Verification items for the finished model (mm, model axes). Round coordinates to 2 decimals unless told otherwise and drop trailing zeros. Order: outer loops, then holes, each group sorted by start corner. A loop starts at its lowest first (then second) coordinate and runs counter-clockwise, first axis right, second up. Notation, with made-up numbers: (36, -18) -> (78, -18) arc R22 cw to (78, 20) -> close; hole circle Ø10 at (88.25, -34). An arc over 180 degrees is marked (long way). Return JSON: item names as keys, results as strings. Group by question number.
Item 1: Draft check along Y on faces 1 (the flat face through (9, 0, 9)), 2 (the cylindrical face through (8.628, 7.255, 8.124)), 3 (the flat face through (0, 11, 9)). Enter one of: pulls with the +Y half, pulls with the -Y half, needs draft (parallel to the pull), parting line crosses it, or undercut.
Item 2: Sectioned sample at C-C on y = 6. Record the cut outline in (x, z).
Item 3: Depth check by flat-ended pin: pin 1 Ø8 at (x, y) = (8, 5) entering from -Z; pin 2 Ø3 at (y, z) = (8.78, 8.76) entering from -X. Enter the tip coordinate at first touch or a pass-through.
Item 4: Sectioned sample at B-B on x = 7.25. Record the cut outline in (y, z), plus the area to 3 significant figures.
Item 5: Sectioned sample at D-D on y = 3.5. Record the cut outline in (x, z).
Item 6: Scan lines: probe 1 along Z at (x, y) = (16.5, 7.5) (3 decimals); probe 2 along Z at (x, y) = (2.25, 7.75); probe 3 along Y at (x, z) = (9, 9.25). Record each from-to range of solid material in increasing order. Write a range as from..to.
Item 7: Sectioned sample at A-A on z = 9.25. Record the cut outline in (x, y).
Autodesk Fusion 360 part; units mm, degrees
sketch "Sketch1" plane through (0, 0, 0) normal (0, 0, 1) x (1, 0, 0)
  line L0 (0, 0) -> (17.5, 0)
  line L1 (17.5, 0) -> (17.5, 17.5)
  line L2 (17.5, 17.5) -> (0, 17.5)
  line L3 (0, 17.5) -> (0, 0)
  dimension "d1" = 17.5
  dimension "d2" = 17.5
extrude "Extrude1" add sketch "Sketch1" along normal blind 17.5
sketch "Sketch2" plane through (0, 0, 0) normal (-1, 0, 0) x (0, -1, 0)
  line L0 (-17.5, 0) -> (0, 0)
  line L1 (0, 0) -> (0, 17.5)
  line L2 (0, 17.5) -> (-17.5, 17.5)
  line L3 (-17.5, 17.5) -> (-17.5, 0)
  circle A0 centre (-8.7787, 8.7562) radius 8.7563
  circle A1 centre (-8.7787, 8.7562) radius 1.65
  dimension "d5" = 3.3
extrude "Extrude2" cut sketch "Sketch2" against normal blind 33 contours A1
chamfer "Chamfer1" distance 1 distance2 12 1 edges at (8.75, 0, 0) measured on face at (5.8333, 0, 5.8333)
Recorded:
{
 "1": {"face 1": "pulls with the -Y half", "face 2": "undercut", "face 3": "needs draft"},
 "2": {"outline": "(0, 0.5) -> (17.5, 0.5) -> (17.5, 17.5) -> (0, 17.5) -> close"},
 "3": {"pin 1": "z = 0.25", "pin 2": "through"},
 "4": {"outline": "(0, 1) -> (12, 0) -> (17.5, 0) -> (17.5, 17.5) -> (0, 17.5) -> close; hole circle Ø3.3 at (8.78, 8.76)", "area": "292 mm²"},
 "5": {"outline": "(0, 0.71) -> (17.5, 0.71) -> (17.5, 17.5) -> (0, 17.5) -> close"},
 "6": {"probe 1": "0.375..7.713, 9.799..17.5", "probe 2": "0.35..7.47, 10.05..17.5", "probe 3": "0..7.2, 10.35..17.5"},
 "7": {"outline": "(0, 0) -> (17.5, 0) -> (17.5, 7.2) -> (0, 7.2) -> close; (0, 10.35) -> (17.5, 10.35) -> (17.5, 17.5) -> (0, 17.5) -> close"}
}
